Work out the finished part from the listing and answer in its coordinate system (mm). A direction names the side the tool comes from. Coordinates: 2 decimals unless noted, no trailing zeros. Write each loop counter-clockwise with the first axis right and the second up, starting at its lowest first coordinate (ties: lowest second). Pieces come first, ordered by that corner, then holes. Notation, with made-up numbers: M -24,-0.5 L 4,-0.5 A24 ccw 4,10.5 Z; hole C 84.5,44 d10. An arc over 180 degrees is marked long. Use CSV: the item, a comma, the result in double quotes.
from build123d import *

# Parameters (mm, degrees)
SKETCH1_R           = 400
BOSS_EXTRUDE1_DEPTH = 10
BOSS_EXTRUDE5_DEPTH = 130
BOSS_EXTRUDE6_START = -30
SKETCH1_4_R         = 400
BOSS_EXTRUDE6_DEPTH = 30
SKETCH4_W           = 162.910444241
SKETCH4_H           = 350.538335194
BOSS_EXTRUDE7_DEPTH = 450


with BuildPart() as part:
    # Sketch1 → Boss-Extrude1 (new body)
    with BuildSketch(Plane(origin=(0, 0, 0), x_dir=(1, 0, 0), z_dir=(0, 1, 0))):
        with Locations(Location((0, 0, 0), (0, 0, 270))):
            Circle(SKETCH1_R)
    extrude(amount=BOSS_EXTRUDE1_DEPTH)

    # Sketch3 → Boss-Extrude5 (add)
    with BuildSketch(Plane(origin=(0, 10, 0), x_dir=(1, 0, 0), z_dir=(0, 1, 0))):
        with BuildLine():
            Line((-4.6, -30.015), (4.6, -30.015))
            Line((4.6, -30.015), (4.6, -24.573156085))
            ThreePointArc((4.6, -24.573156085), (0, 25), (-4.6, -24.573156085))
            Line((-4.6, -24.573156085), (-4.6, -30.015))
        make_face()
    extrude(amount=BOSS_EXTRUDE5_DEPTH)

    # Sketch1_4 → Boss-Extrude6 (add)
    with BuildSketch(Plane(origin=(0, 0, 0), x_dir=(1, 0, 0), z_dir=(0, 1, 0)).offset(BOSS_EXTRUDE6_START)):
        with Locations(Location((0, 0, 0), (0, 0, 270))):
            Circle(SKETCH1_4_R)
    extrude(amount=BOSS_EXTRUDE6_DEPTH)

    # Sketch4 → Boss-Extrude7 (add)
    with BuildSketch(Plane.XZ.offset(30)):
        with Locations((-117.407871884, -47.749612967)):
            Rectangle(SKETCH4_W, SKETCH4_H)
    extrude(amount=BOSS_EXTRUDE7_DEPTH)


solid = part.part
Item 1: Consider probe 1 along Y at (x, z) = (97.5, 317.5); probe 2 along X at (y, z) = (-271, -110.5); probe 3 along Y at (x, z) = (-196.5, -162). Determine where each line is inside the solid, lowest interval first.
Answer:
probe 1,"y = -30 to 10"
probe 2,"x = -198.86 to -35.95"
probe 3,"y = -480 to 10"
Item 2: The part is cut by section D-D (y = -15). Write down the section's boundary in (x, z).
Answer:
outline,"C 0,0 d800"
Item 3: A tool of negligible diameter and unlimited length cuts with its end or side. For faces 1 (the face through (-119, -252, -223.019)), 2 (the face through (-119, -252, 127.52)), 3 (the face through (-198.863, -252, -50)), 4 (the face through (1.03, 74.09, -24.98)), 5 (the face through (-35.953, -252, -50)), from which of +Z, -Z, +X, -X, +Y, -Y can it reach the whole face along a straight path? Write none if from no direction.
Answer:
face 1,"-Z, +X, -X, -Y"
face 2,"+Z, +X, -X, -Y"
face 3,"+Z, -Z, -X, -Y"
face 4,"+Y"
face 5,"+Z, -Z, +X, -Y"
Item 4: The part is cut by section C-C (x = 48). Write down the section's boundary in (y, z).
Answer:
outline,"M -30,-397.11 L 10,-397.11 L 10,397.11 L -30,397.11 Z"
Item 5: Given pin 1 (4.5 mm diameter, centred on y = 88.5, z = 27, fed in from -X); pin 2 (8 mm diameter, centred on y = -299, z = -131, fed in from +X); pin 3 (5 mm diameter, centred on x = -131, z = -15.5, fed in from +Y), each flat-ended and moving along its own axis, determine where each tip first touches the part or whether it passes through.
Answer:
pin 1,"stops at x = -4.6"
pin 2,"stops at x = -35.95"
pin 3,"stops at y = 10"
Item 6: The part is cut by section B-B (y = -421). Write down the section's boundary in (x, z).
Answer:
outline,"M -198.86,-223.02 L -35.95,-223.02 L -35.95,127.52 L -198.86,127.52 Z"
Item 7: The part is cut by section A-A (z = 0). Write down the section's boundary in (x, y).
Answer:
outline,"M -400,-30 L -198.86,-30 L -198.86,-480 L -35.95,-480 L -35.95,-30 L 400,-30 L 400,10 L 25,10 L 25,140 L -25,140 L -25,10 L -400,10 Z"
